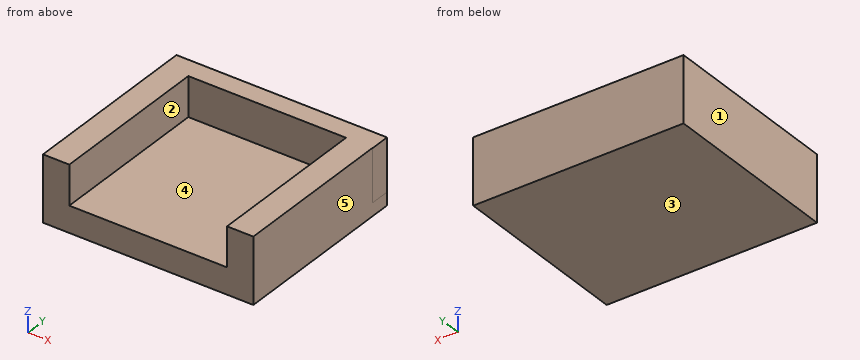
from build123d import *

# Parameters (mm, degrees)
F0_W     = 25.4
F0_H     = 25.4
F0_W_2   = 152.4
F0_H_2   = 38.1
F1_DEPTH = 177.8
F2_W     = 203.2
F2_H     = 19.2293866986
F3_DEPTH = 50.8


# Not quite as in the source:
# - a feature names something its author has since deleted; it is built from what else it names


with BuildPart() as f1:
    # F0 (on Front) → F1 (new body)
    with BuildSketch(Plane.XZ):
        with Locations((-88.9, 0)):
            Rectangle(F0_W, F0_H)
        Rectangle(F0_W_2, F0_H)
        with Locations((88.9, 0)):
            Rectangle(F0_W, F0_H)
        with Locations((88.9, 31.75)):
            Rectangle(F0_W, F0_H_2)
        with Locations((-88.9, 31.75)):
            Rectangle(F0_W, F0_H_2)
    extrude(amount=F1_DEPTH)

    # F2 (on Top) → F3 (join)
    with BuildSketch(Plane.XY):
        with Locations((0.2353874207, -9.6146933493)):
            Rectangle(F2_W, F2_H)
    extrude(amount=F3_DEPTH)


solid = f1.part
Could you check a few things on this model? Use its own coordinates, in mm. Face numbers are marked on the shaded views. A direction names the side the tool comes from. Round coordinates to 2 decimals unless told otherwise and drop trailing zeros. Order: outer loops, then holes, each group sorted by start corner. A loop starts at its lowest first (then second) coordinate and runs counter-clockwise, first axis right, second up.
(1) Please list where these lines run through material, in increasing order: line 1 along X through (y, z) = (-33.5, 17); line 2 along Y through (x, z) = (14.5, 14.5); line 3 along X through (y, z) = (-124.5, 10).
Response values:
line 1: x = -101.6 to -76.2, 76.2 to 101.6
line 2: y = -19.23 to 0
line 3: x = -101.6 to 101.6
(2) Imagine slicing it at C-C (x = 42.5). Write out the boundary of the cut face in (y, z).
Response values:
outline: (-177.8, -12.7) - (0, -12.7) - (0, 50.8) - (-19.23, 50.8) - (-19.23, 12.7) - (-177.8, 12.7) - close
(3) Imagine slicing it at A-A (y = -46). Write out the boundary of the cut face in (x, z).
Response values:
outline: (-101.6, -12.7) - (101.6, -12.7) - (101.6, 50.8) - (76.2, 50.8) - (76.2, 12.7) - (-76.2, 12.7) - (-76.2, 50.8) - (-101.6, 50.8) - close
(4) Which directions (+Z, -Z, +X, -X, +Y, -Y) give clear straight access to the entire face, cutting with the end or side of a thin tool? Please do the marked faces 1 and 2.
Response values:
face 1: +Z, -Z, -X, +Y, -Y
face 2: +Z, -Y
(5) If we mould it in two halves opening along X, with no side actions, what happens to the marked faces 3, 4 and 5? For each: released by +X, released by -X, zero draft, split by the parting line, or undercut.
Response values:
face 3: zero draft
face 4: undercut
face 5: released by +X
(6) I'm going to push flat-ended pins straight in: pin 1 (12 mm diameter, centred on y = -61.5, z = 17.5, fed in from +X); pin 2 (6 mm diameter, centred on x = 6.5, y = -78.5, fed in from +Z). Where does each tip first touch, or does it pass through?
Response values:
pin 1: stops at x = 101.6
pin 2: stops at z = 12.7
(7) Imagine slicing it at B-B (z = 38). Write out the boundary of the cut face in (x, y), plus the area to 3 significant figures.
Response values:
outline: (-101.6, -177.8) - (-76.2, -177.8) - (-76.2, -19.23) - (76.2, -19.23) - (76.2, -177.8) - (101.6, -177.8) - (101.6, -19.23) - (101.84, -19.23) - (101.84, 0) - (-101.6, 0) - close
area: 12,000 mm2
